Design review of the part built by this model. Coordinates are the model's own, in mm. Coordinates: 2 decimals unless noted, no trailing zeros. Write each loop counter-clockwise with the first axis right and the second up, starting at its lowest first coordinate (ties: lowest second). Pieces come first, ordered by that corner, then holes.
Q1. For probe 1 along Y at (x, z) = (-0.1, 2.9); probe 2 along Y at (x, z) = (0, 1.6); probe 3 along Y at (x, z) = (1.65, 0.75), list the stretches that pass through material, from the lowest coordinate up.
Q2. Take a section at A-A (x = 0). Give the boundary of the cut face in (y, z) (3 decimals).
Q3. Mouldability with a two-part tool opening along X and no side actions: class faces 1 (the flat face through (0, 34.493, 2)), 2 (the cylindrical face through (-0.198, -2.883, 1.565)), 3 (the flat face through (-2.286, 15, 2)) as pulls with the +X half, pulls with the -X half, needs draft (parallel to the pull), parting line crosses it, or undercut.
Q4. Take a section at B-B (z = 0.5). Give the boundary of the cut face in (x, y) (1 decimal).
Autodesk Inventor part; units mm, degrees
ref_plane "YZ Plane" through (0, 0, 0) normal (1, 0, 0) x (0, 1, 0)
ref_plane "XZ Plane" through (0, 0, 0) normal (0, 1, 0) x (-1, 0, 0)
ref_plane "XY Plane" through (0, 0, 0) normal (0, 0, 1) x (1, 0, 0)
sketch "Sketch1" plane through (0, 0, 0) normal (0, 0, 1) x (1, 0, 0)
  line L0 (-2.286, -3.4798) -> (2.286, -3.4798)
  line L1 (-2.286, -3.4798) -> (-2.286, 33.3502)
  line L2 (-2.286, 33.3502) -> (2.286, 33.3502)
  line L3 (2.286, 33.3502) -> (2.286, -3.4798)
  line L4 (2.286, 14.9352) -> (-2.286, 14.9352)
  line L5 (0, 33.3502) -> (0, 31.242)
  circle A0 centre (0, 31.242) radius 1.524
  circle A1 centre (0, -1.3716) radius 1.524
  line L6 (0, -3.4798) -> (0, -4.6228)
  line L7 (0, -4.6228) -> (2.286, -4.6228)
  line L8 (2.286, -4.6228) -> (2.286, -3.4798)
  line L9 (-2.286, -3.4798) -> (-2.286, -4.6228)
  line L10 (-2.286, -4.6228) -> (0, -4.6228)
  line L11 (0, 34.4932) -> (2.286, 34.4932)
  line L12 (2.286, 34.4932) -> (2.286, 33.3502)
  line L13 (-2.286, 33.3502) -> (-2.286, 34.4932)
  line L14 (-2.286, 34.4932) -> (0, 34.4932)
  point P0 (0, 0)
  dimension "d0" = 4.572
  dimension "d1" = 36.83
  dimension "d2" = 2.1082
  dimension "d3" = 3.048
  dimension "d7" = 1.143
extrude "Extrusion1" add sketch "Sketch1" along normal blind 3.175
fillet "Fillet2" radius 1.5875 4 edges at (2.286, 34.4932, 1.5875) (-2.286, 34.4932, 1.5875) (-2.286, -4.6228, 1.5875) (2.286, -4.6228, 1.5875)
properties part number "hank - linkage"
Response:
1. probe 1: y = -4.62 to -2.89, 0.15 to 29.72, 32.76 to 34.49
1. probe 2: y = -4.62 to -2.9, 0.15 to 29.72, 32.77 to 34.49
1. probe 3: y = -4.31 to 34.18
2. outline: (-4.623, 0) - (-2.896, 0) - (-2.896, 3.175) - (-4.623, 3.175) - close; (0.152, 0) - (29.718, 0) - (29.718, 3.175) - (0.152, 3.175) - close; (32.766, 0) - (34.493, 0) - (34.493, 3.175) - (32.766, 3.175) - close
3. face 1: needs draft
3. face 2: undercut
3. face 3: pulls with the -X half
4. outline: (-2.3, -3) arc R1.6 ccw to (-0.7, -4.6) - (0.7, -4.6) arc R1.6 ccw to (2.3, -3) - (2.3, 32.9) arc R1.6 ccw to (0.7, 34.5) - (-0.7, 34.5) arc R1.6 ccw to (-2.3, 32.9) - close; hole circle Ø3 at (0, -1.4); hole circle Ø3 at (0, 31.2)
